Build history of the part. All positions in model axes, mm. Face numbers are marked on the shaded views. A direction names the side the tool comes from. Give positions to 0.01 mm unless a question says otherwise; leave off trailing zeros. Write each loop counter-clockwise with the first axis right and the second up, starting at its lowest first coordinate (ties: lowest second). Pieces come first, ordered by that corner, then holes. Notation, with made-up numbers: M 36.25,53.5 L 41.25,53.5 A37 ccw 41.25,92.5 Z; hole C 89.25,-35.5 d10. An arc over 180 degrees is marked long. Return JSON: item names as keys, results as strings. Group by question number.
Q1. Flat gauge pins, fed straight in: pin 1 Ø0.9 at (x, y) = (4.5, 2.5) entering from -Z; pin 2 Ø4 at (y, z) = (5, 10) entering from -X; pin 3 Ø0.6 at (x, y) = (-1, -4.5) entering from +Z; pin 4 Ø5 at (x, y) = (4.5, 4.5) entering from +Z. Where does each tip first touch, or does it go through?
Q2. Wall check: probe 1 along X at (y, z) = (-1.25, 15.25); probe 2 along Y at (x, z) = (1.5, 15.75) (3 decimals); probe 3 along X at (y, z) = (0, 2.75). Give the ranges that are in metal, low to high.
Q3. Band-saw the part on A-A, the plane x = 0. Give the cut face in (y, z) (1 decimal), then the cut area to 3 significant figures.
Q4. Tool access for the marked faces 1, 2 and 3: list every direction of +Z, -Z, +X, -X, +Y, -Y with a clear straight run to the whole face (end or side of a thin tool).
Q5. Band-saw the part on B-B, the plane y = 0. Give the cut face in (x, z), then the cut area to 3 significant figures.
Q6. Band-saw the part on D-D, the plane y = -4. Give the cut face in (x, z), then the cut area to 3 significant figures.
Q7. Band-saw the part on C-C, the plane z = 18.75. Give the cut face in (x, y) (3 decimals), then the cut area to 3 significant figures.
Q8. Pull direction Z, two halves, no side cores. Call the marked faces 4, 5 and 6: +Z half, -Z half, draft (parallel to the pull), parting line (faces both ways), or undercut.
from build123d import *

# Parameters (mm, degrees)
SKETCH2_W           = 10.16
SKETCH2_H           = 6.35
BOSS_EXTRUDE1_DEPTH = 16.256


with BuildPart() as part:
    # Sketch1 → Revolve1 (revolve)
    with BuildSketch(Plane(origin=(0, 0, 0), x_dir=(1, 0, 0), z_dir=(0, 1, 0))):
        with BuildLine():
            Line((0, 6.20395), (0, -4.3688))
            Line((0, -4.3688), (-5.3086, -4.3688))
            Line((-5.3086, -4.3688), (-5.3086, -0.4826))
            Line((-5.3086, -0.4826), (-6.9215, -0.4826))
            Line((-6.9215, -0.4826), (-6.9215, 0))
            Line((-6.9215, 0), (-6.20395, 0))
            ThreePointArc((-6.20395, 0), (-4.386855115, 4.386855115), (0, 6.20395))
        make_face()
    revolve(axis=Axis((0, 0, -6.20395), (0, 0, 1)))

    # Sketch2 → Boss-Extrude1 (add)
    with BuildSketch(Plane.XY.offset(4.3688)):
        Rectangle(SKETCH2_W, SKETCH2_H)
    extrude(amount=BOSS_EXTRUDE1_DEPTH)


solid = part.part
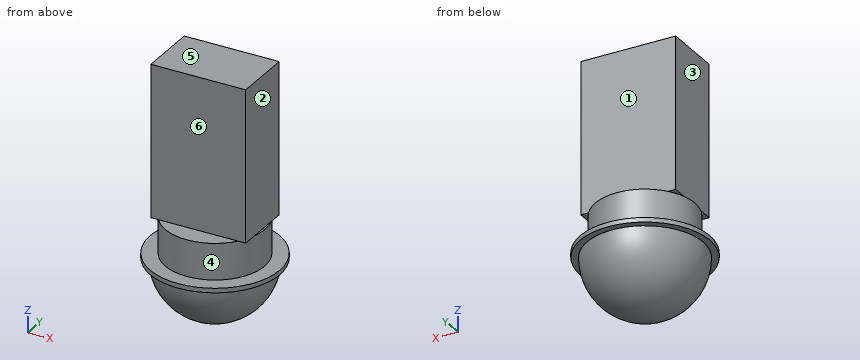
From the geometry:
{
 "1": {"pin 1": "stops at z = -4.05", "pin 2": "stops at x = -5.08", "pin 3": "stops at z = 4.37", "pin 4": "stops at z = 20.62"},
 "2": {"probe 1": "x = -5.08 to 5.08", "probe 2": "y = -3.175 to 3.175", "probe 3": "x = -5.31 to 5.31"},
 "3": {"outline": "M -6.9,0 L -6.2,0 A6.2 ccw 6.2,0 L 6.9,0 L 6.9,0.5 L 5.3,0.5 L 5.3,4.4 L 3.2,4.4 L 3.2,20.6 L -3.2,20.6 L -3.2,4.4 L -5.3,4.4 L -5.3,0.5 L -6.9,0.5 Z", "area": "212 mm^2"},
 "4": {"face 1": "+Z, +X, -X, +Y", "face 2": "+Z, +X, +Y, -Y", "face 3": "+Z, -X, +Y, -Y"},
 "5": {"outline": "M -6.92,0 L -6.2,0 A6.2 ccw 6.2,0 L 6.92,0 L 6.92,0.48 L 5.31,0.48 L 5.31,4.37 L 5.08,4.37 L 5.08,20.62 L -5.08,20.62 L -5.08,4.37 L -5.31,4.37 L -5.31,0.48 L -6.92,0.48 Z", "area": "274 mm^2"},
 "6": {"outline": "M -5.65,0 L -4.74,0 A4.74 ccw 4.74,0 L 5.65,0 L 5.65,0.48 L 3.49,0.48 L 3.49,4.37 L -3.49,4.37 L -3.49,0.48 L -5.65,0.48 Z", "area": "67.9 mm^2"},
 "7": {"outline": "M -5.08,-3.175 L 5.08,-3.175 L 5.08,3.175 L -5.08,3.175 Z", "area": "64.5 mm^2"},
 "8": {"face 4": "undercut", "face 5": "+Z half", "face 6": "draft"}
}
